```python
from build123d import *

# Parameters (mm, degrees)
F0_R     = 8
F1_DEPTH = 10
F2_R     = 5
F3_DEPTH = 7
F4_R     = 0.5
F5_DEPTH = 25
F6_R     = 0.5
F7_DEPTH = 25


with BuildPart() as f1:
    # F0 (on Top) → F1 (new body)
    with BuildSketch(Plane.XY):
        Circle(F0_R)
    extrude(amount=F1_DEPTH)

    # F2 (on face) → F3 (join)
    with BuildSketch(Plane(origin=(0, 0, 0), x_dir=(1, 0, 0), z_dir=(0, 0, -1))):
        Circle(F2_R)
    extrude(amount=F3_DEPTH)

    # F4 (on Right) → F5 (cut)
    with BuildSketch(Plane.YZ):
        with Locations((0, -4)):
            Circle(F4_R)
    extrude(amount=-F5_DEPTH, mode=Mode.SUBTRACT)

    # F6 (on face) → F7 (cut)
    with BuildSketch(Plane(origin=(0, 0, 0), x_dir=(0, -1, 0), z_dir=(-1, 0, 0))):
        with Locations((0, -4)):
            Circle(F6_R)
    extrude(amount=-F7_DEPTH, mode=Mode.SUBTRACT)


solid = f1.part
```
Verification items for the finished model (mm, model axes). A direction names the side the tool comes from. Coordinates: 2 decimals unless noted, no trailing zeros. Write each loop counter-clockwise with the first axis right and the second up, starting at its lowest first coordinate (ties: lowest second). Pieces come first, ordered by that corner, then holes. Notation, with made-up numbers: M 4.25,35 L 36.25,35 A20 ccw 36.25,51 Z; hole C 60.5,-19.75 d3. An arc over 180 degrees is marked long. Answer as a JSON object with one key per item and string values. Group by question number.
(1) Cross-section at A-A, the plane y = 0. Record the cut outline in (x, z), and give its area (3 significant figures).
(2) Tool access check on faces 1 (the face through (5.2, 0.1, 0)), 2 (the face through (0, 0, 10)). Record the directions out of +Z, -Z, +X, -X, +Y, -Y that give a thin tool (end or side, any length) a straight path to the whole face; none if there is none.
(3) Material ranges on line 1 (Z direction, x = -3.7, y = 0); line 2 (Z direction, x = -5.5, y = 5.75); line 3 (X direction, y = 0.25, z = 3.75), recorded low to high.
(4) Cross-section at D-D, the plane y = -3. Record the cut outline in (x, z), and give its area (3 significant figures).
(5) Gauge pin test, flat ends, axial feed: pin 1 (1.5 mm diameter, centred on y = 2, z = 3.5, fed in from +X); pin 2 (1 mm diameter, centred on y = -4.5, z = 1, fed in from -X); pin 3 (3 mm diameter, centred on y = -3, z = -2.5, fed in from -X). Record the tip position at first contact, or that the pin passes through.
(6) Cross-section at B-B, the plane x = -2.25. Record the cut outline in (y, z), and give its area (3 significant figures).
Reply:
{
 "1": {"outline": "M -8,0 L -5,0 L -5,-3.5 L 5,-3.5 L 5,0 L 8,0 L 8,10 L -8,10 Z; M -5,-7 L 5,-7 L 5,-4.5 L -5,-4.5 Z", "area": "220 mm²"},
 "2": {"face 1": "-Z", "face 2": "+Z, +X, -X, +Y, -Y"},
 "3": {"line 1": "-7 to -4.5, -3.5 to 10", "line 2": "0 to 10", "line 3": "-8 to 8"},
 "4": {"outline": "M -7.42,0 L -4,0 L -4,-7 L 4,-7 L 4,0 L 7.42,0 L 7.42,10 L -7.42,10 Z", "area": "204 mm²"},
 "5": {"pin 1": "x = 7.9", "pin 2": "x = -6.93", "pin 3": "x = -4.77"},
 "6": {"outline": "M -7.68,0 L -4.47,0 L -4.47,-7 L 4.47,-7 L 4.47,0 L 7.68,0 L 7.68,10 L -7.68,10 Z; hole C 0,-4 d1", "area": "215 mm²"}
}
